Read the model definition and answer for the solid it produces. Units are mm, in the model's axes. Coordinates: 2 decimals unless noted, no trailing zeros. Order: outer loops, then holes, each group sorted by start corner. A loop starts at its lowest first (then second) coordinate and runs counter-clockwise, first axis right, second up. Notation, with made-up numbers: (16.5, -3.5) - (30.5, -3.5) arc R30 ccw to (30.5, 25.5) - close; hole circle Ø11 at (62, -27.5). An arc over 180 degrees is marked (long way). Use one line per item in the form item = value.
```python
from build123d import *

# Parameters (mm, degrees)
ESTRUSIONE_ESTRUSIONE1_DEPTH = 2
ESTRUSIONE_ESTRUSIONE2_DEPTH = 2


with BuildPart() as part:
    # Schizzo1 → Estrusione-Estrusione1 (new body)
    with BuildSketch(Plane(origin=(0, 0, 0), x_dir=(1, 0, 0), z_dir=(0, 1, 0))):
        with BuildLine():
            Line((5, 0), (61, 0))
            ThreePointArc((61, 0), (64.535533906, 1.464466094), (66, 5))
            Line((66, 5), (66, 80))
            ThreePointArc((66, 80), (64.535533906, 83.535533906), (61, 85))
            Line((61, 85), (5, 85))
            ThreePointArc((5, 85), (1.464466094, 83.535533906), (0, 80))
            Line((0, 80), (0, 5))
            ThreePointArc((0, 5), (1.464466094, 1.464466094), (5, 0))
        make_face()
    extrude(amount=ESTRUSIONE_ESTRUSIONE1_DEPTH)

    # Schizzo2 → Estrusione-Estrusione2 (add)
    with BuildSketch(Plane.XZ):
        with BuildLine():
            Line((60.393923704, -83.5), (5.606076296, -83.5))
            ThreePointArc((5.606076296, -83.5), (2.702641903, -82.297358097), (1.5, -79.393923704))
            Line((1.5, -79.393923704), (1.5, -5.606076296))
            ThreePointArc((1.5, -5.606076296), (2.702641903, -2.702641903), (5.606076296, -1.5))
            Line((5.606076296, -1.5), (60.393923704, -1.5))
            ThreePointArc((60.393923704, -1.5), (63.297358097, -2.702641903), (64.5, -5.606076296))
            Line((64.5, -5.606076296), (64.5, -79.393923704))
            ThreePointArc((64.5, -79.393923704), (63.297358097, -82.297358097), (60.393923704, -83.5))
        make_face()
    extrude(amount=ESTRUSIONE_ESTRUSIONE2_DEPTH)


solid = part.part
```
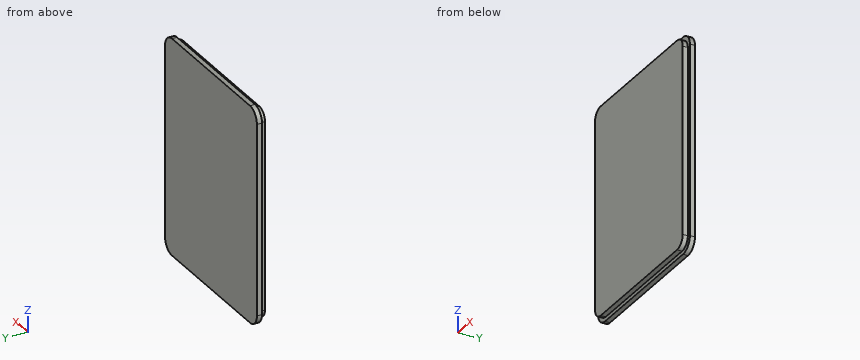
(1) Given pin 1 Ø1 at (y, z) = (-1.5, -54.5) entering from +X; pin 2 Ø0.6 at (x, y) = (40.5, -0.5) entering from +Z; pin 3 Ø0.6 at (y, z) = (-1, -61) entering from -X, each flat-ended and moving along its own axis, determine where each tip first touches the part or whether it passes through.
Answer list:
pin_1 = 64.5
pin_2 = -1.5
pin_3 = 1.5
(2) Straight lines are drawn through the part: L1, parallel to Z at x = 16.5, y = -0.85; L2, parallel to X at y = -1.2, z = -43.5; L3, parallel to X at y = 1.3, z = -4. For each, find the intervals that lie inside material, in ascending order.
Answer list:
L1 = -83.5 to -1.5
L2 = 1.5 to 64.5
L3 = 0.1 to 65.9
(3) Section B-B, the plane x = 23.5 is taken. Write down the section's boundary in (y, z).
Answer list:
outline = (-2, -83.5) - (0, -83.5) - (0, -85) - (2, -85) - (2, 0) - (0, 0) - (0, -1.5) - (-2, -1.5) - close
(4) Section A-A, the plane z = -22 is taken. Write down the section's boundary in (x, y), then the cut area to 3 significant figures.
Answer list:
outline = (0, 0) - (1.5, 0) - (1.5, -2) - (64.5, -2) - (64.5, 0) - (66, 0) - (66, 2) - (0, 2) - close
area = 258 mm2
